Geometry check sheet. Reference: drawing and pictorial views, mm from the part's lowest x, y, z. A direction names the side the tool comes from. Round coordinates to 2 decimals unless told otherwise and drop trailing zeros. Order: outer loops, then holes, each group sorted by start corner. A loop starts at its lowest first (then second) coordinate and runs counter-clockwise, first axis right, second up.
(1) Thickness scan on probe 1 along Z at (x, y) = (34, 3.5) (1 decimal); probe 2 along Y at (x, z) = (36, 20); probe 3 along X at (y, z) = (5, 21). Record the ranges inside material, lowest first.
(2) Sectioned sample at D-D, the plane x = 48. Enter the section's corners in (y, z), and give its area (3 significant figures).
(3) Tool access check on the marked faces 4 and 5. Record the directions out of +Z, -Z, +X, -X, +Y, -Y that give a thin tool (end or side, any length) a straight path to the whole face; none if there is none.
(4) Sectioned sample at A-A, the plane y = 5.5. Enter the section's corners in (x, z), and give its area (3 significant figures).
(5) Depth check by flat-ended pin: pin 1 (10.5 mm diameter, centred on x = 31.5, z = 25.5, fed in from +Y); pin 2 (4 mm diameter, centred on x = 36, y = 5.5, fed in from +Z) (1 decimal); pin 3 (5 mm diameter, centred on x = 18, y = 7.5, fed in from +Z). Enter the tip coordinate at first touch or a pass-through.
(6) Sectioned sample at C-C, the plane z = 27.5. Enter the section's corners in (x, y), and give its area (3 significant figures).
(7) Sectioned sample at B-B, the plane x = 36. Enter the section's corners in (y, z) (1 decimal).
(8) Mould release check, pull along X, two halves, no side actions. Record for the marked faces 1, 2 and 3: released by +X, released by -X, zero draft, split by the parting line, or undercut.
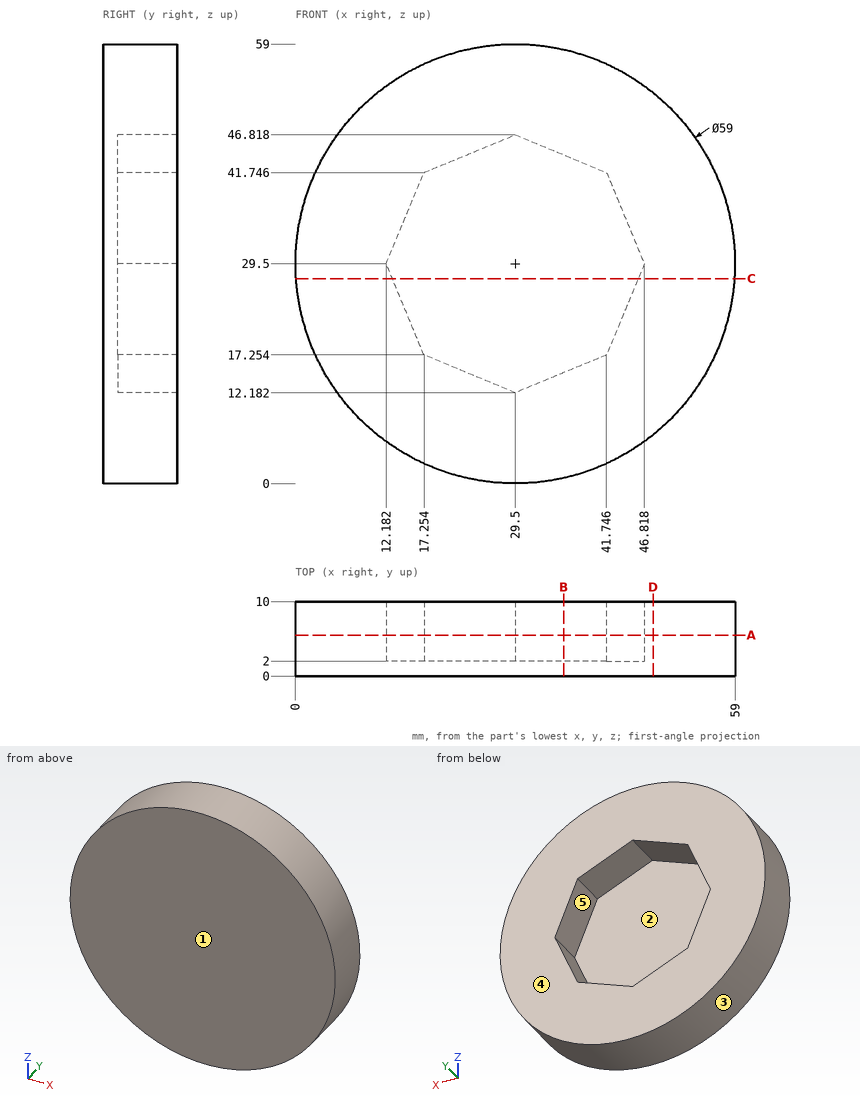
Derived:
1. probe 1: z = 0.3 to 14, 45 to 58.7
1. probe 2: y = 0 to 2
1. probe 3: x = 1.25 to 15.7, 43.3 to 57.75
2. outline: (0, 6.52) - (10, 6.52) - (10, 52.48) - (0, 52.48) - close
2. area: 460 mm2
3. face 4: +Z, -Z, +X, -X, +Y
3. face 5: +Y
4. outline: circle Ø59 at (29.5, 29.5); hole (12.18, 29.5) - (17.25, 17.25) - (29.5, 12.18) - (41.75, 17.25) - (46.82, 29.5) - (41.75, 41.75) - (29.5, 46.82) - (17.25, 41.75) - close
4. area: 1,890 mm2
5. pin 1: stops at y = 2
5. pin 2: stops at z = 58.7
5. pin 3: stops at z = 57.59
6. outline: (0.07, 0) - (58.93, 0) - (58.93, 10) - (45.99, 10) - (45.99, 2) - (13.01, 2) - (13.01, 10) - (0.07, 10) - close
6. area: 325 mm2
7. outline: (0, 0.7) - (10, 0.7) - (10, 14.9) - (2, 14.9) - (2, 44.1) - (10, 44.1) - (10, 58.3) - (0, 58.3) - close
8. face 1: zero draft
8. face 2: undercut
8. face 3: split by the parting line
